Read the model definition and answer for the solid it produces. Units are mm, in the model's axes. Round coordinates to 2 decimals unless told otherwise and drop trailing zeros. Loops run counter-clockwise (first coordinate to the right, second up) from the corner with the lowest first, then second, coordinate; pieces in that order, holes last. Notation, with made-up numbers: (43.5, -18.5) -> (99.5, -18.5) arc R7 cw to (99.5, -6.5) -> close; hole circle Ø9 at (84.25, -11). An arc over 180 degrees is marked (long way). Put each result on its own line as item: value.
from build123d import *

# Parameters (mm, degrees)
BOSS_EXTRUDE1_DEPTH              = 3.175
F_17_64_0_26563_DIAMETER_HOLE1_D = 6.747002
SKETCH5_W                        = 254
SKETCH5_H                        = 38.1
CUT_EXTRUDE1_DEPTH               = 916.815527617
FILLET1_R                        = 3.175


with BuildPart() as part:
    # Sketch1 → Boss-Extrude1 (new body)
    with BuildSketch(Plane(origin=(0, 0, 0), x_dir=(1, 0, 0), z_dir=(0, 1, 0))):
        with BuildLine():
            Line((-717.55, 504.825), (-717.55, 392.610512242))
            ThreePointArc((-717.55, 392.610512242), (-718.516729937, 387.750432651), (-721.269743879, 383.630256121))
            Line((-721.269743879, 383.630256121), (-761.07006403, 343.82993597))
            ThreePointArc((-761.07006403, 343.82993597), (-761.758317516, 342.799891837), (-762, 341.584871939))
            Line((-762, 341.584871939), (-762, -504.825))
            ThreePointArc((-762, -504.825), (-761.07006403, -507.07006403), (-758.825, -508))
            Line((-758.825, -508), (758.825, -508))
            ThreePointArc((758.825, -508), (761.07006403, -507.07006403), (762, -504.825))
            Line((762, -504.825), (762, 341.584871939))
            ThreePointArc((762, 341.584871939), (761.758317516, 342.799891837), (761.07006403, 343.82993597))
            Line((761.07006403, 343.82993597), (721.269743879, 383.630256121))
            ThreePointArc((721.269743879, 383.630256121), (718.516729937, 387.750432651), (717.55, 392.610512242))
            Line((717.55, 392.610512242), (717.55, 504.825))
            ThreePointArc((717.55, 504.825), (716.62006403, 507.07006403), (714.375, 508))
            Line((714.375, 508), (-714.375, 508))
            ThreePointArc((-714.375, 508), (-716.62006403, 507.07006403), (-717.55, 504.825))
        make_face()
    extrude(amount=BOSS_EXTRUDE1_DEPTH)

    # 17/64 (0.26563) Diameter Hole1 (through all)
    with Locations(Plane(origin=(0, 3.175, 0), x_dir=(1, 0, 0), z_dir=(0, 1, 0))):
        with Locations((-565.15, 422.275), (565.15, 422.275), (565.15, -269.875), (-565.15, -269.875), (-682.625, 127), (-447.675, 127), (-682.625, -107.95), (-447.675, -107.95), (-117.475, 127), (117.475, 127), (-117.475, -107.95), (117.475, -107.95), (447.675, 127), (682.625, 127), (447.675, -107.95), (682.625, -107.95)):
            Hole(F_17_64_0_26563_DIAMETER_HOLE1_D / 2)

    # Sketch5 → Cut-Extrude1 (cut, through all)
    with BuildSketch(Plane(origin=(0, 3.175, 0), x_dir=(1, 0, 0), z_dir=(0, 1, 0))):
        with Locations((0, -488.95)):
            Rectangle(SKETCH5_W, SKETCH5_H)
    extrude(amount=-CUT_EXTRUDE1_DEPTH, mode=Mode.SUBTRACT)

    # Fillet1
    fillet1_edges = [part.edges().sort_by_distance(p)[0] for p in [
        (-127, 1.5875, 508),
        (-127, 1.5875, 469.9),
        (127, 1.5875, 469.9),
        (127, 1.5875, 508),
    ]]
    fillet(fillet1_edges, radius=FILLET1_R)


solid = part.part
Item 1: Flat-ended cylindrical pins translate along their axes: pin 1 Ø1 at (y, z) = (1.5, -466) entering from -X; pin 2 Ø5.5 at (x, z) = (682.625, -127) entering from +Y; pin 3 Ø1 at (y, z) = (2, -457) entering from +X; pin 4 Ø1 at (x, y) = (4.5, 1) entering from +Z. Find the tip coordinate at first contact, or state that the pin passes through.
Derived:
pin 1: stops at x = -717.55
pin 2: passes through
pin 3: stops at x = 717.55
pin 4: stops at z = 469.9
Item 2: The part is cut by section A-A (x = 70). Determine the outline of the cut face in (y, z) (3 decimals).
Derived:
outline: (0, -508) -> (3.175, -508) -> (3.175, 469.9) -> (0, 469.9) -> close
Item 3: Find the intervals of material crossed by line 1 along Z through (x, y) = (8, 1.9), in increasing order.
Derived:
line 1: z = -508 to 469.9
